Read the model definition and answer for the solid it produces. Units are mm, in the model's axes. Face numbers are marked on the shaded views. A direction names the side the tool comes from. Give positions to 0.01 mm unless a question says otherwise; leave off trailing zeros. Write each loop counter-clockwise with the first axis right and the second up, starting at its lowest first coordinate (ties: lowest second). Pieces come first, ordered by that corner, then holes. Notation, with made-up numbers: (49, 53) -> (103, 53) arc R14 ccw to (103, 77) -> close; hole circle Ø11 at (-15, -36.5). An arc over 180 degrees is marked (long way). Answer as CSV lines item,"result". Start each with the question number.
1. The part is cut by section A-A, the plane x = 174. Determine the outline of the cut face in (y, z), and give its area (3 significant figures).
2. Given pin 1 (8 mm diameter, centred on x = 87, z = -83, fed in from +Y); pin 2 (3.5 mm diameter, centred on x = 138, z = -1, fed in from -Y); pin 3 (4 mm diameter, centred on x = 128.5, z = -29.5, fed in from -Y), each flat-ended and moving along its own axis, determine where each tip first touches the part or whether it passes through.
3. The part is cut by section D-D, the plane z = -179. Determine the outline of the cut face in (x, y).
4. Find the intervals of material crossed by line 1 (Y direction, x = 47.5, z = -86.5); line 2 (Y direction, x = 189.5, z = -87), in increasing order.
5. The part is cut by section C-C, the plane y = 25.5. Give the number of separate pieces and of enclosed holes in the cut face, and give its area (3 significant figures).
6. The part is cut by section B-B, the plane y = 6.5. Determine the outline of the cut face in (x, z), and give its area (3 significant figures).
7. A tool of negligible diameter and unlimited length cuts with its end or side. For the marked faces 1 and 2, from which of +Z, -Z, +X, -X, +Y, -Y can it reach the whole face along a straight path? Write none if from no direction.
from build123d import *

# Parameters (mm, degrees)
BOSS_EXTRUDE2_DEPTH = 300
SKETCH3_R           = 5
BOSS_EXTRUDE3_DEPTH = 10


with BuildPart() as part:
    # Sketch2 → Boss-Extrude2 (new body)
    with BuildSketch(Plane(origin=(0, 0, 0), x_dir=(0, 0, -1), z_dir=(1, 0, 0))):
        with BuildLine():
            Line((195.359179423, -2.939387691), (3, 36.325765386))
            Line((3, 36.325765386), (3, 0))
            Line((3, 0), (0, 0))
            Line((0, 0), (0, 36.325765386))
            ThreePointArc((0, 36.325765386), (1.102633404, 38.649555394), (3.6, 39.265153077))
            Line((3.6, 39.265153077), (195.959179423, 0))
            Line((195.959179423, 0), (195.359179423, -2.939387691))
        make_face()
    extrude(amount=BOSS_EXTRUDE2_DEPTH)

    # Sketch3 → Boss-Extrude3 (add)
    with BuildSketch(Plane(origin=(0, 38.4, -7.838367177), x_dir=(1, 0, 0), z_dir=(0, 0.9797958971132714, -0.19999999999999998))):
        with Locations(Location((53.264501209, 93.837117307, 0), (0, 0, 90))):
            Circle(SKETCH3_R)
        with Locations(Location((143.264501209, 93.837117307, 0), (0, 0, 90))):
            Circle(SKETCH3_R)
        with Locations(Location((233.264501209, 93.837117307, 0), (0, 0, 90))):
            Circle(SKETCH3_R)
    extrude(amount=BOSS_EXTRUDE3_DEPTH)


solid = part.part
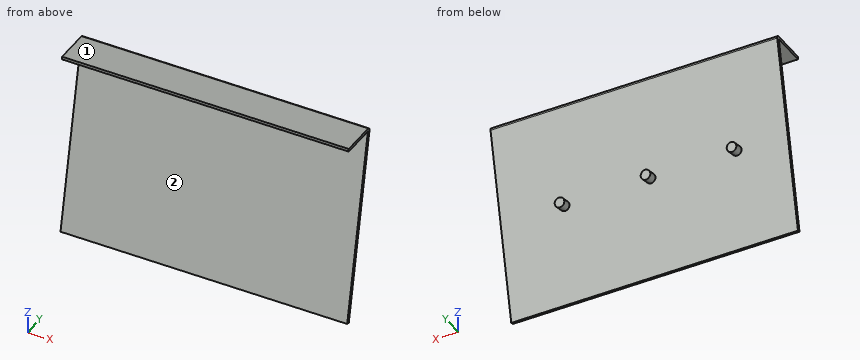
Results found:
1,outline,"(-2.94, -195.36) -> (0, -195.96) -> (39.27, -3.6) arc R3 ccw to (36.33, 0) -> (0, 0) -> (0, -3) -> (36.33, -3) -> close"
1,area,"706 mm²"
2,pin 1,"stops at y = 23.87"
2,pin 2,"stops at y = 0"
2,pin 3,"stops at y = 30.51"
3,outline,"(0, 0.4) -> (300, 0.4) -> (300, 3.46) -> (0, 3.46) -> close"
4,line 1,"y = 19.28 to 22.34"
4,line 2,"y = 19.18 to 22.24"
5,separate pieces,"5"
5,enclosed holes,"0"
5,area,"5,640 mm²"
6,outline,"(0, -164.12) -> (300, -164.12) -> (300, -149.12) -> (0, -149.12) -> close; (0, -3) -> (300, -3) -> (300, 0) -> (0, 0) -> close"
6,area,"5,400 mm²"
7,face 1,"+Z, +X, -X, +Y, -Y"
7,face 2,"+X, -X, -Y"
